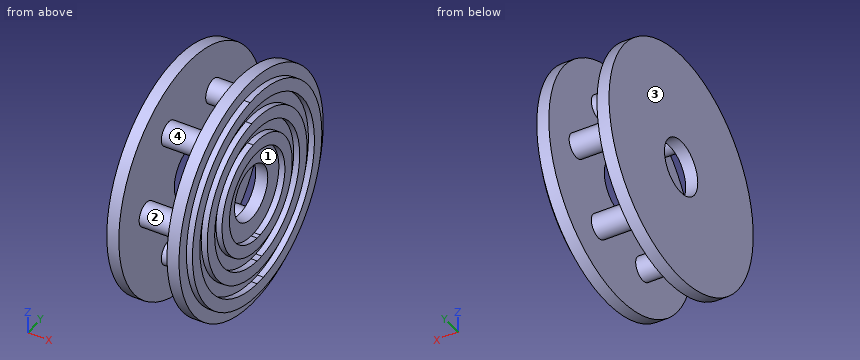
```python
from build123d import *

# Parameters (mm, degrees)
SKETCH1_R           = 9.75
SKETCH1_R_2         = 2.25
BOSS_EXTRUDE1_DEPTH = 1
BOSS_EXTRUDE2_DEPTH = 0.5
SKETCH3_R           = 1
BOSS_EXTRUDE3_DEPTH = 4
SKETCH4_R           = 9.75
SKETCH4_R_2         = 2.25
BOSS_EXTRUDE4_DEPTH = 1


with BuildPart() as part:
    # Sketch1 → Boss-Extrude1 (new body)
    with BuildSketch(Plane(origin=(0, 0, 0), x_dir=(0, 0, -1), z_dir=(1, 0, 0))):
        Circle(SKETCH1_R)
        Circle(SKETCH1_R_2, mode=Mode.SUBTRACT)
    extrude(amount=BOSS_EXTRUDE1_DEPTH)

    # Sketch2 → Boss-Extrude2 (add)
    with BuildSketch(Plane(origin=(1, 0, 0), x_dir=(0, 0, -1), z_dir=(1, 0, 0))):
        with BuildLine():
            ThreePointArc((8.696853314, 0.96293428), (-0.96293428, 8.696853314), (-8.696853314, -0.96293428))
            ThreePointArc((-8.696853314, -0.96293428), (0.482199906, -8.736703226), (8.75, 0))
            ThreePointArc((8.75, 0), (8.736703226, 0.482199906), (8.696853314, 0.96293428))
        make_face()
        with BuildLine():
            ThreePointArc((7.75, 0), (0.427091345, -7.738222857), (-7.702927221, -0.852884648))
            ThreePointArc((-7.702927221, -0.852884648), (-0.852884648, 7.702927221), (7.702927221, 0.852884648))
            ThreePointArc((7.702927221, 0.852884648), (7.738222857, 0.427091345), (7.75, 0))
        make_face(mode=Mode.SUBTRACT)
        with BuildLine():
            ThreePointArc((6.709001128, 0.742835016), (-0.742835016, 6.709001128), (-6.709001128, -0.742835016))
            ThreePointArc((-6.709001128, -0.742835016), (0.371982785, -6.739742488), (6.75, 0))
            ThreePointArc((6.75, 0), (6.739742488, 0.371982785), (6.709001128, 0.742835016))
        make_face()
        with BuildLine():
            ThreePointArc((5.75, 0), (0.316874224, -5.74126212), (-5.715075035, -0.632785384))
            ThreePointArc((-5.715075035, -0.632785384), (-0.632785384, 5.715075035), (5.715075035, 0.632785384))
            ThreePointArc((5.715075035, 0.632785384), (5.74126212, 0.316874224), (5.75, 0))
        make_face(mode=Mode.SUBTRACT)
        with BuildLine():
            ThreePointArc((4.721148942, 0.522735752), (-0.522735752, 4.721148942), (-4.721148942, -0.522735752))
            ThreePointArc((-4.721148942, -0.522735752), (0.261765663, -4.742781751), (4.75, 0))
            ThreePointArc((4.75, 0), (4.742781751, 0.261765663), (4.721148942, 0.522735752))
        make_face()
        with BuildLine():
            ThreePointArc((3.75, 0), (0.206657103, -3.744301382), (-3.727222849, -0.41268612))
            ThreePointArc((-3.727222849, -0.41268612), (-0.41268612, 3.727222849), (3.727222849, 0.41268612))
            ThreePointArc((3.727222849, 0.41268612), (3.744301382, 0.206657103), (3.75, 0))
        make_face(mode=Mode.SUBTRACT)
    extrude(amount=BOSS_EXTRUDE2_DEPTH)

    # Sketch3 → Boss-Extrude3 (add)
    with BuildSketch(Plane.ZY):
        with Locations((0, 6)):
            Circle(SKETCH3_R)
        with Locations((5.196152423, 3)):
            Circle(SKETCH3_R)
        with Locations((5.196152423, -3)):
            Circle(SKETCH3_R)
        with Locations((0, -6)):
            Circle(SKETCH3_R)
        with Locations((-5.196152423, -3)):
            Circle(SKETCH3_R)
        with Locations((-5.196152423, 3)):
            Circle(SKETCH3_R)
    extrude(amount=BOSS_EXTRUDE3_DEPTH)

    # Sketch4 → Boss-Extrude4 (add)
    with BuildSketch(Plane.ZY.offset(4)):
        Circle(SKETCH4_R)
        Circle(SKETCH4_R_2, mode=Mode.SUBTRACT)
    extrude(amount=BOSS_EXTRUDE4_DEPTH)


solid = part.part
```
Geometry: final body of the model. Coordinates: model frame, mm. Face numbers are marked on the shaded views. A direction names the side the tool comes from. Round coordinates to 2 decimals unless told otherwise and drop trailing zeros. Write each loop counter-clockwise with the first axis right and the second up, starting at its lowest first coordinate (ties: lowest second). Pieces come first, ordered by that corner, then holes.
Item 1: Pin query (flat end, axial travel): P1, Ø4, axis at y = 0, z = 0, coming from the +X side; P2, Ø10, axis at y = 0, z = -2, coming from the +X side; P3, Ø2, axis at x = 0.5, y = 6.5, coming from the -Z side; P4, Ø2, axis at x = -2.5, y = 2, coming from the +Z side. Return the tip coordinate at first contact, or that it passes through.
Item 2: Set-up query: the marked faces 1 and 2. Return all of +Z, -Z, +X, -X, +Y, -Y with unobstructed straight access to the full face (end or side cutting, diameter ignored); none if empty.
Item 3: Section query D-D (y = -6.25). Return loops of the section in (x, z), plus the area to 3 significant figures.
Item 4: Section query B-B (x = -3). Return loops of the section in (y, z), plus the area to 3 significant figures.
Item 5: Mould query, pull axis Y, two halves, no side actions, for the marked faces 3 and 4. Classes: +Y half, -Y half, draft (parallel to the pull), parting line (faces both ways), or undercut.
Item 6: Section query A-A (y = 7.25). Return loops of the section in (x, z).
Item 7: Material intervals for L1, parallel to X at y = 4.75, z = -6; L2, parallel to X at y = -7.5, z = -4.25; L3, parallel to Y at x = -4.5, z = 0, sorted ascending.
Completed:
1. P1: passes through
1. P2: stops at x = 1.5
1. P3: stops at z = -8.05
1. P4: stops at z = 6.2
2. face 1: +X
2. face 2: none
3. outline: (-5, -7.48) - (-4, -7.48) - (-4, -0.97) - (0, -0.97) - (0, -7.48) - (1, -7.48) - (1, -6.12) - (1.5, -6.12) - (1.5, -4.58) - (1, -4.58) - (1, -2.55) - (1.5, -2.55) - (1.5, 2.55) - (1, 2.55) - (1, 4.58) - (1.5, 4.58) - (1.5, 6.12) - (1, 6.12) - (1, 7.48) - (0, 7.48) - (0, 0.97) - (-4, 0.97) - (-4, 7.48) - (-5, 7.48) - close
3. area: 41.8 mm2
4. outline: circle Ø2 at (-6, 0); circle Ø2 at (-3, -5.2); circle Ø2 at (-3, 5.2); circle Ø2 at (3, -5.2); circle Ø2 at (3, 5.2); circle Ø2 at (6, 0)
4. area: 18.8 mm2
5. face 3: draft
5. face 4: undercut
6. outline: (-5, -6.52) - (-4, -6.52) - (-4, 6.52) - (-5, 6.52) - close; (0, -6.52) - (1, -6.52) - (1, -4.9) - (1.5, -4.9) - (1.5, -2.74) - (1, -2.74) - (1, 2.74) - (1.5, 2.74) - (1.5, 4.9) - (1, 4.9) - (1, 6.52) - (0, 6.52) - close
7. L1: x = -5 to -4, 0 to 1
7. L2: x = -5 to -4, 0 to 1.5
7. L3: y = -9.75 to -2.25, 2.25 to 9.75
